Can you work these out from the model? Positions are in its coordinate system, mm. A direction names the side the tool comes from. Give positions to 0.01 mm unless a question says otherwise; leave off trailing zeros. Write each loop counter-clockwise with the first axis right and the second up, starting at its lowest first coordinate (ties: lowest second). Pieces come first, ordered by that corner, then holes.
1. Suppose I cut it at A-A (x = 132). Please give me the cut outline in (y, z), and give its area (3 significant figures).
2. Suppose I cut it at C-C (x = 64.5). Please give me the cut outline in (y, z), and give its area (3 significant figures).
3. Suppose I cut it at B-B (z = 6.25). Give the number of separate pieces and of enclosed holes in the cut face, and give its area (3 significant figures).
4. Thinking about a two-plate mould opening in Y: for faces 1 (the cylindrical face through (119.061, 2.854, 6.93)), 2 (the flat face through (76, 11, 6)), 3 (the flat face through (165, 0, 6)), which applies, pulls with the +Y half, pulls with the -Y half, needs draft (parallel to the pull), parting line crosses it, or undercut?
5. If I drill on probe 1 along Z at (x, y) = (33, -2.75); probe 2 along Y at (x, z) = (44, 8); probe 3 along Y at (x, z) = (64, 1), over which ranges is the centre line in solid material (lowest first)?
6. I'm going to push a flat-ended pin straight in: pin 1 (4 mm diameter, centred on x = 113.5, y = 3, fed in from +Z). Where does the tip first touch, or does it pass through?
7. On a 3-axis mill with a long thin cutter (end or side, diameter ignored), from which of +Z, -Z, +X, -X, +Y, -Y can I reach the whole of each face in a straight line? I mean faces 4 (the flat face through (77, 0, 2.2)), 5 (the flat face through (76, 0, 0)), 6 (the flat face through (78, 0, 2)), 7 (the cylindrical face through (97.061, 2.854, 6.93)), 8 (the flat face through (76, -11, 6)). Say none if no direction works.
```python
from build123d import *

# Parameters (mm, degrees)
F0_W     = 22
F0_H     = 22
F0_W_2   = 8
F0_H_2   = 8
F1_DEPTH = 2
F2_W     = 176
F2_H     = 22
F2_R     = 9.5
F3_DEPTH = 10
F4_W     = 8
F4_H     = 0.2
F5_DEPTH = 176.001


with BuildPart() as f1:
    # F0 (on Top) → F1 (new body)
    with BuildSketch(Plane.XY):
        Rectangle(F0_W, F0_H)
        Rectangle(F0_W_2, F0_H_2, mode=Mode.SUBTRACT)
        with Locations((22, 0)):
            Rectangle(F0_W, F0_H)
        with Locations((22, 0)):
            Rectangle(F0_W_2, F0_H_2, mode=Mode.SUBTRACT)
        with Locations((44, 0)):
            Rectangle(F0_W, F0_H)
        with Locations((44, 0)):
            Rectangle(F0_W_2, F0_H_2, mode=Mode.SUBTRACT)
        with Locations((66, 0)):
            Rectangle(F0_W, F0_H)
        with Locations((66, 0)):
            Rectangle(F0_W_2, F0_H_2, mode=Mode.SUBTRACT)
        with Locations((88, 0)):
            Rectangle(F0_W, F0_H)
        with Locations((88, 0)):
            Rectangle(F0_W_2, F0_H_2, mode=Mode.SUBTRACT)
        with Locations((110, 0)):
            Rectangle(F0_W, F0_H)
        with Locations((110, 0)):
            Rectangle(F0_W_2, F0_H_2, mode=Mode.SUBTRACT)
        with Locations((132, 0)):
            Rectangle(F0_W, F0_H)
        with Locations((132, 0)):
            Rectangle(F0_W_2, F0_H_2, mode=Mode.SUBTRACT)
        with Locations((154, 0)):
            Rectangle(F0_W, F0_H)
        with Locations((154, 0)):
            Rectangle(F0_W_2, F0_H_2, mode=Mode.SUBTRACT)
    extrude(amount=F1_DEPTH)

    # F2 (on face) → F3 (join)
    with BuildSketch(Plane.XY.offset(2)):
        with Locations((77, 0)):
            Rectangle(F2_W, F2_H)
        Circle(F2_R, mode=Mode.SUBTRACT)
        with Locations((22, 0)):
            Circle(F2_R, mode=Mode.SUBTRACT)
        with Locations((44, 0)):
            Circle(F2_R, mode=Mode.SUBTRACT)
        with Locations((66, 0)):
            Circle(F2_R, mode=Mode.SUBTRACT)
        with Locations((88, 0)):
            Circle(F2_R, mode=Mode.SUBTRACT)
        with Locations((110, 0)):
            Circle(F2_R, mode=Mode.SUBTRACT)
        with Locations((132, 0)):
            Circle(F2_R, mode=Mode.SUBTRACT)
        with Locations((154, 0)):
            Circle(F2_R, mode=Mode.SUBTRACT)
    extrude(amount=F3_DEPTH)

    # F4 (on face) → F5 (cut, through all)
    with BuildSketch(Plane.YZ.offset(165)):
        with Locations((0, 2.1)):
            Rectangle(F4_W, F4_H)
    extrude(amount=-F5_DEPTH, mode=Mode.SUBTRACT)


solid = f1.part
```
Checks:
1. outline: (-11, 0) - (-4, 0) - (-4, 2) - (-9.5, 2) - (-9.5, 12) - (-11, 12) - close; (4, 0) - (11, 0) - (11, 12) - (9.5, 12) - (9.5, 2) - (4, 2) - close
1. area: 58.0 mm2
2. outline: (-11, 0) - (-4, 0) - (-4, 2) - (-9.38, 2) - (-9.38, 12) - (-11, 12) - close; (4, 0) - (11, 0) - (11, 12) - (9.38, 12) - (9.38, 2) - (4, 2) - close
2. area: 60.4 mm2
3. separate pieces: 1
3. enclosed holes: 8
3. area: 1,600 mm2
4. face 1: undercut
4. face 2: pulls with the +Y half
4. face 3: needs draft
5. probe 1: z = 0 to 2, 2.2 to 12
5. probe 2: y = -11 to -9.5, 9.5 to 11
5. probe 3: y = -11 to -4, 4 to 11
6. pin 1: stops at z = 2
7. face 4: +X, -X
7. face 5: -Z, +X, -X, +Y, -Y
7. face 6: none
7. face 7: +Z
7. face 8: +Z, -Z, +X, -X, -Y
